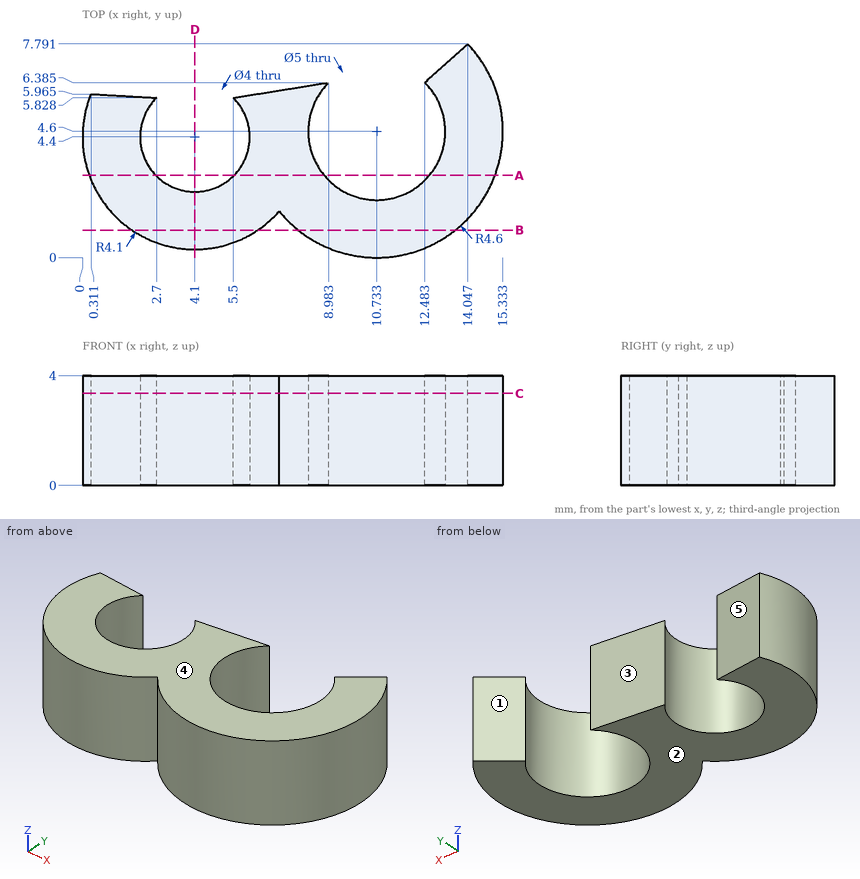
Job drawing, mm, ordinate dimensions from the low corner. One solid piece. A direction names the side the tool comes from. Give positions to 0.01 mm unless a question says otherwise; leave off trailing zeros. Order: outer loops, then holes, each group sorted by start corner. A loop starts at its lowest first (then second) coordinate and runs counter-clockwise, first axis right, second up. Notation, with made-up numbers: M -20,41.5 L -1,41.5 A12 ccw -1,56.5 Z; hole C 10,15.5 d4. An arc over 180 degrees is marked long. Put each result on its own line as item: value. Start each with the question number.
(1) Band-saw the part on B-B on y = 1. Give the cut face in (x, z).
(2) Pull direction X, two halves, no side cores. Call the marked faces 1, 2 and 3: released by +X, released by -X, zero draft, split by the parting line, or undercut.
(3) Band-saw the part on D-D on x = 4.1. Give the cut face in (y, z).
(4) Pin check, flat tips, straight feed: pin 1 Ø1.5 at (y, z) = (6.5, 2) entering from -X; pin 2 Ø1 at (y, z) = (7, 1) entering from -X; pin 3 Ø1.5 at (y, z) = (1.5, 1.5) entering from +X. Stop position of each tip, or through.
(5) Drill centre lines: L1, parallel to X at y = 4.6, z = 2.65 (1 decimal); L2, parallel to X at y = 5.25, z = 1.95; L3, parallel to X at y = 1, z = 1.1 (1 decimal). Where is each one in solid material? Low to high. Write a range as [from, to].
(6) Band-saw the part on C-C on z = 3.35. Give the cut face in (x, y) (1 decimal).
(7) Tool access for the marked faces 4 and 5: list every direction of +Z, -Z, +X, -X, +Y, -Y with a clear straight run to the whole face (end or side of a thin tool).
(8) Band-saw the part on A-A on y = 3. Give the cut face in (x, z) (1 decimal), then the cut area to 3 significant figures.
Results below:
1. outline: M 1.81,0 L 6.39,0 L 6.39,4 L 1.81,4 Z; M 7.87,0 L 13.6,0 L 13.6,4 L 7.87,4 Z
2. face 1: released by -X
2. face 2: zero draft
2. face 3: undercut
3. outline: M 0.3,0 L 2.4,0 L 2.4,4 L 0.3,4 Z
4. pin 1: stops at x = 0.23
4. pin 2: stops at x = 12.61
4. pin 3: stops at x = 14.69
5. L1: x = [0, 2.1], [6.1, 8.2], [13.2, 15.3]
5. L2: x = [0.09, 2.29], [5.91, 8.32], [13.15, 15.29]
5. L3: x = [1.8, 6.4], [7.9, 13.6]
6. outline: M 0.3,6 A4.1 ccw 7.2,1.7 A4.6 ccw long 14,7.8 L 12.5,6.4 A2.5 cw long 9,6.4 L 5.5,5.8 A2 cw long 2.7,5.8 Z
7. face 4: +Z, +X, -X, +Y, -Y
7. face 5: +Z, -Z, +Y
8. outline: M 0.2,0 L 2.7,0 L 2.7,4 L 0.2,4 Z; M 5.5,0 L 8.8,0 L 8.8,4 L 5.5,4 Z; M 12.7,0 L 15,0 L 15,4 L 12.7,4 Z
8. area: 32.4 mm2
